Source: three-view drawing plus pictorial views. Frame: mm from the lowest corner of the part. Round coordinates to 2 decimals unless told otherwise and drop trailing zeros. Order: outer loops, then holes, each group sorted by start corner. A loop starts at its lowest first (then second) coordinate and runs counter-clockwise, first axis right, second up. Notation, with made-up numbers: M 30.25,31.25 L 41.25,31.25 A9 cw 41.25,39.25 Z; hole C 58.5,38.25 d2. An arc over 180 degrees is marked long. Return JSON: item names as keys, results as strings. Group by question number.
Q1. Contact query for flat-ended pins moving along their axis: pin 1 (2 mm diameter, centred on x = 43, z = 2, fed in from -Y); pin 2 (2 mm diameter, centred on x = 46, z = 1, fed in from -Y); pin 3 (2 mm diameter, centred on x = 24, y = 220, fed in from -Z); pin 4 (2 mm diameter, centred on x = 35.5, z = 2.5, fed in from +Y). Output: stop coordinate, or through.
Q2. Cut plane A-A on y = 21. Output: boundary loops of the cut face in (x, z), and give its area (3 significant figures).
Q3. Ray query, probe 1 along X at (y, z) = (153, 0.8); probe 2 along Y at (x, z) = (38, 2.8). Return the intervals inside material, ascending.
Q4. Cut plane B-B on x = 11. Output: boundary loops of the cut face in (y, z).
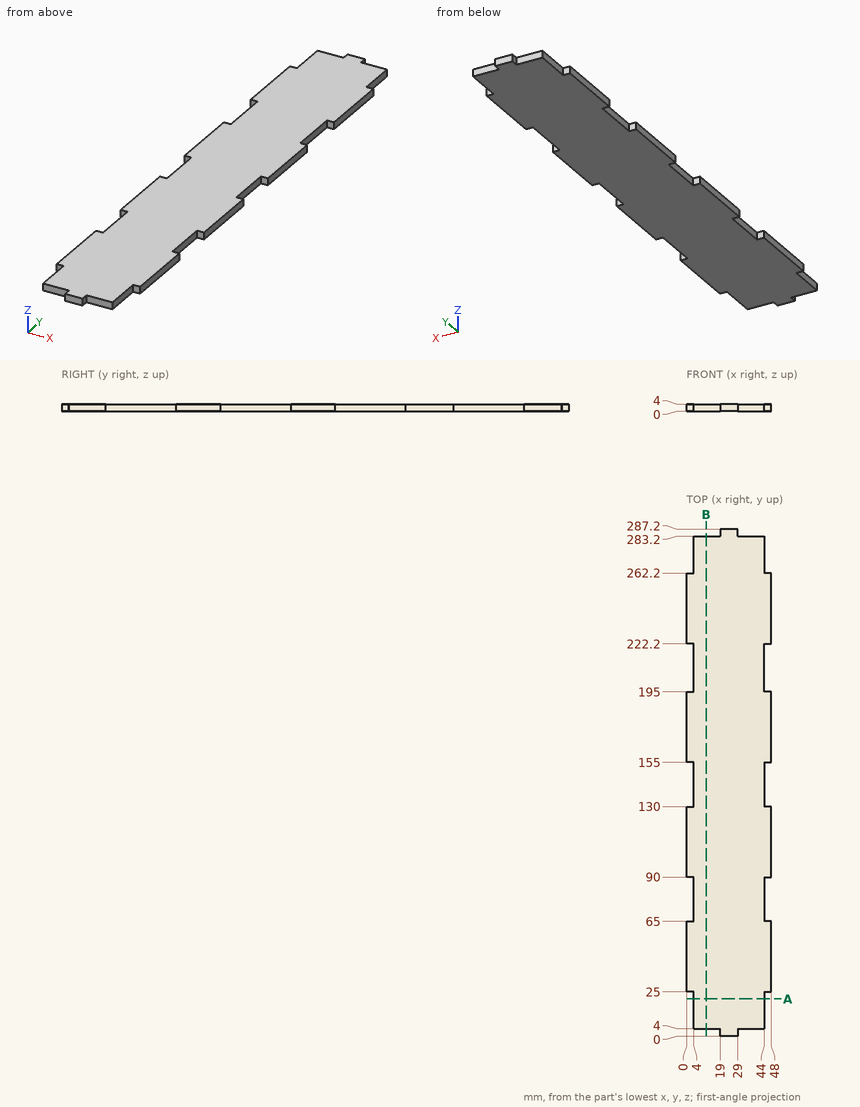
Result sheet:
{
 "1": {"pin 1": "stops at y = 4", "pin 2": "stops at y = 25", "pin 3": "stops at z = 0", "pin 4": "stops at y = 283.2"},
 "2": {"outline": "M 4,0 L 44,0 L 44,4 L 4,4 Z", "area": "160 mm²"},
 "3": {"probe 1": "x = 4 to 44", "probe 2": "y = 4 to 283.2"},
 "4": {"outline": "M 4,0 L 283.2,0 L 283.2,4 L 4,4 Z"}
}
